Build history of the part. All positions in model axes, mm. A direction names the side the tool comes from. Give positions to 0.01 mm unless a question says otherwise; leave off trailing zeros. Write each loop counter-clockwise with the first axis right and the second up, starting at its lowest first coordinate (ties: lowest second). Pieces come first, ordered by that corner, then holes. Notation, with made-up numbers: (22.25, -35.75) -> (51.25, -35.75) arc R21 cw to (51.25, -5.75) -> close; hole circle Ø5 at (52.25, 52). An arc over 180 degrees is marked (long way). Put each result on its own line as item: value.
from build123d import *
from build123d.topology import SkipClean

# Parameters (mm, degrees)
SKETCH1_R           = 9.5
BOSS_EXTRUDE1_DEPTH = 200
BOSS_EXTRUDE2_START = -70
SKETCH2_R           = 30
SKETCH2_R_2         = 9.5
BOSS_EXTRUDE2_DEPTH = 70
CUT_EXTRUDE1_DEPTH  = 137.747943312
CIRPATTERN1_COUNT   = 3


with BuildPart() as part:
    # Sketch1 → Boss-Extrude1 (new body)
    with BuildSketch(Plane(origin=(0, 0, 0), x_dir=(1, 0, 0), z_dir=(0, 1, 0))):
        with Locations(Location((0, 0, 0), (0, 0, 270))):
            Circle(SKETCH1_R)
    extrude(amount=BOSS_EXTRUDE1_DEPTH)

    # Sketch2 → Boss-Extrude2 (add)
    with BuildSketch(Plane(origin=(0, 200, 0), x_dir=(1, 0, 0), z_dir=(0, 1, 0)).offset(BOSS_EXTRUDE2_START)):
        with Locations(Location((0, 0, 0), (0, 0, 270))):
            Circle(SKETCH2_R)
        with Locations(Location((0, 0, 0), (0, 0, 270))):
            Circle(SKETCH2_R_2, mode=Mode.SUBTRACT)
    extrude(amount=BOSS_EXTRUDE2_DEPTH)

    # Sketch3 → Cut-Extrude1 (cut, through all)
    with SkipClean():  # the faces are left unmerged after this step: merging them gives an invalid solid
        with BuildSketch(Plane.XZ.offset(-130)):
            with BuildLine():
                Line((20.805356407, -37.93850618), (-20.805356407, -37.93850618))
                Line((-20.805356407, -37.93850618), (-3.621476876, -8.782647963))
                ThreePointArc((-3.621476876, -8.782647963), (0, -9.5), (3.621476876, -8.782647963))
                Line((3.621476876, -8.782647963), (20.805356407, -37.93850618))
            make_face()
        cut_extrude1 = extrude(amount=-CUT_EXTRUDE1_DEPTH, mode=Mode.SUBTRACT)

    # CirPattern1: Cut-Extrude1 ×3 about axis
    with SkipClean():  # the faces are left unmerged after this step: merging them gives an invalid solid
        cirpattern1_axis = Axis((0, 0, 0), (0, 1, 0))
        for i in range(1, CIRPATTERN1_COUNT):
            add(cut_extrude1.rotate(cirpattern1_axis, i * 360 / CIRPATTERN1_COUNT), mode=Mode.SUBTRACT)


solid = part.part
1) Slice it at C-C (y = 45). Write the cut outline in (x, z), plus the area to 3 significant figures.
Filled sheet:
outline: circle Ø19 at (0, 0)
area: 284 mm2
2) Slice it at A-A (y = 166). Write the cut outline in (x, z).
Filled sheet:
outline: (-29.98, 1.07) arc R30 ccw to (-14.06, -26.5) -> (-3.62, -8.78) arc R9.5 ccw to (3.62, -8.78) -> (14.06, -26.5) arc R30 ccw to (29.98, 1.07) -> (9.42, 1.26) arc R9.5 ccw to (5.8, 7.53) -> (15.92, 25.43) arc R30 ccw to (-15.92, 25.43) -> (-5.8, 7.53) arc R9.5 ccw to (-9.42, 1.26) -> close
3) Pin check, flat tips, straight feed: pin 1 (2 mm diameter, centred on x = -2.5, y = 119, fed in from -Z); pin 2 (8 mm diameter, centred on y = 141.5, z = 4.5, fed in from +X); pin 3 (8 mm diameter, centred on x = -23, z = -10.5, fed in from -Y). Stop position of each tip, or through.
Filled sheet:
pin 1: z = -9.38
pin 2: x = 30
pin 3: y = 130
4) Wall check: L1, parallel to Z at x = -7.5, y = 23; L2, parallel to Y at x = 4.5, z = 9; L3, parallel to Z at x = 11, y = 177. Give the ranges that are in metal, low to high.
Filled sheet:
L1: -5.83 to 5.83
L2: 130 to 200
L3: -21.3 to 1.24, 16.73 to 27.91
5) Pull direction Z, two halves, no side cores. Call faces 4 (the cylindrical face through (0, 165, 30)), 5 (the flat face through (0, 0, 0)), 6 (the flat face through (8.77, 164.51, -17.52)), 7 (the flat face through (10.786, 164.51, 16.353)): released by +Z, released by -Z, zero draft, split by the parting line, or undercut.
Filled sheet:
face 4: released by +Z
face 5: zero draft
face 6: released by -Z
face 7: undercut
6) Slice it at D-D (x = -22). Write the cut outline in (y, z).
Filled sheet:
outline: (130, -20.4) -> (200, -20.4) -> (200, 1.14) -> (130, 1.14) -> close
7) Tool access for faces 1 (the flat face through (-10.927, 164.51, 16.604)), 2 (the flat face through (0, 200, 1)), 3 (the flat face through (-8.92, 164.51, -17.77)): list every direction of +Z, -Z, +X, -X, +Y, -Y with a clear straight run to the whole face (end or side of a thin tool).
Filled sheet:
face 1: -X, +Y, -Y
face 2: +Z, -Z, +X, -X, +Y
face 3: -Z, +Y, -Y
8) Slice it at B-B (x = 0). Write the cut outline in (y, z).
Filled sheet:
outline: (0, -9.5) -> (200, -9.5) -> (200, 30) -> (130, 30) -> (130, 9.5) -> (0, 9.5) -> close
